Autodesk Inventor part; units mm, degrees
ref_plane "YZ Plane" through (0, 0, 0) normal (1, 0, 0) x (0, 1, 0)
ref_plane "XZ Plane" through (0, 0, 0) normal (0, 1, 0) x (-1, 0, 0)
ref_plane "XY Plane" through (0, 0, 0) normal (0, 0, 1) x (1, 0, 0)
sketch "Sketch1" plane through (0, 0, 0) normal (0, 1, 0) x (-1, 0, 0)
  line L0 (0, 0) -> (0, -44) construction
  line L1 (0, -44) -> (-31.9955, -44) construction
  line L2 (-31.9955, -44) -> (-31.9955, 0) construction
  line L3 (-31.9955, 0) -> (0, 0) construction
  dimension "d5" = 44
  dimension "d9" = 31.9955
sketch "Sketch2" plane through (0, 0, 0) normal (0, 1, 0) x (-1, 0, 0)
  line L0 (0, 0) -> (0, -44) construction
  line L1 (0, -44) -> (-31.9955, -44) construction
  line L2 (-31.9955, -44) -> (-31.9955, 0) construction
  line L3 (-31.9955, 0) -> (0, 0) construction
  line L4 (0, 0) -> (-31.9955, 0)
  line L5 (-31.9955, 0) -> (-31.9955, -44)
  line L6 (-31.9955, -44) -> (0, -44)
  line L7 (0, -44) -> (0, 0)
extrude "Extrusion1" add sketch "Sketch2" against normal blind 1.6
decal "Decal1"
sketch "Sketch4" plane through (0, 0, 0) normal (0, 1, 0) x (1, 0, 0)
  line L0 (3.4199, 20.4831) -> (28.4199, 20.4831)
  line L1 (28.4199, 20.4831) -> (28.4199, 40.4831)
  line L2 (28.4199, 40.4831) -> (3.4199, 40.4831)
  line L3 (3.4199, 40.4831) -> (3.4199, 20.4831)
  line L4 (3.4199, 20.4831) -> (28.4199, 40.4831) construction
  line L5 (28.4199, 20.4831) -> (3.4199, 40.4831) construction
  point P0 (0, 0)
  point P1 (15.9199, 30.4831)
  dimension "d14" = 25
  dimension "d15" = 20
hole "Hole1" at (3.4199, 0, -40.4831) at (3.4199, 0, -20.4831) at (28.4199, 0, -20.4831) at (28.4199, 0, -40.4831) direction (0, -1, 0) diameter 3.9 depth 3
properties part number "DFR-08104"
Geometry check sheet. Reference: the model listing, model coordinates, mm. Give positions to 0.01 mm unless a question says otherwise; leave off trailing zeros. Order: outer loops, then holes, each group sorted by start corner. A loop starts at its lowest first (then second) coordinate and runs counter-clockwise, first axis right, second up. Notation, with made-up numbers: M -31.75,16.5 L 14.25,16.5 A28 cw 14.25,39.5 Z; hole C -19.5,36.5 d7. An arc over 180 degrees is marked long. Use a Markdown table: item, result.
Item 1: Draft check along Z on faces 1 (the flat face through (0, -1, -22)), 2 (the cylindrical face through (30.15, -0.81, -19.58)), 3 (the flat face through (16, -1, 0)). Enter one of: +Z half, -Z half, draft (parallel to the pull), parting line (faces both ways), or undercut.
Answers follow:
| item | result |
|---|---|
| face 1 | draft |
| face 2 | undercut |
| face 3 | +Z half |
Item 2: Depth check by flat-ended pin: P1, Ø2.5, axis at x = 28.42, z = -40.48, coming from the +Y side. Enter the tip coordinate at first touch or a pass-through.
Answers follow:
| item | result |
|---|---|
| P1 | passes through |
Item 3: Section check A-A (y = -0.9). Record the cut outline in (x, z), and give its area (3 significant figures).
Answers follow:
| item | result |
|---|---|
| outline | M 0,-44 L 32,-44 L 32,0 L 0,0 Z; hole C 3.42,-40.48 d3.9; hole C 3.42,-20.48 d3.9; hole C 28.42,-40.48 d3.9; hole C 28.42,-20.48 d3.9 |
| area | 1,360 mm2 |
Item 4: Material ranges on line 1 along Z through (x, y) = (3.5, -0.55); line 2 along Z through (x, y) = (28, -0.8); line 3 along X through (y, z) = (-0.1, -40), recorded low to high.
Answers follow:
| item | result |
|---|---|
| line 1 | z = -44 to -42.43, -38.53 to -22.43, -18.53 to 0 |
| line 2 | z = -44 to -42.39, -38.58 to -22.39, -18.58 to 0 |
| line 3 | x = 0 to 1.53, 5.31 to 26.53, 30.31 to 32 |
